Build history of the part. All positions in model axes, mm. Round coordinates to 2 decimals unless told otherwise and drop trailing zeros. Write each loop counter-clockwise with the first axis right and the second up, starting at its lowest first coordinate (ties: lowest second). Pieces come first, ordered by that corner, then holes. Notation, with made-up numbers: (-8.75, 52) - (12.25, 52) arc R23 ccw to (12.25, 82) - close; hole circle Ø6 at (55, -30.5). An arc over 180 degrees is marked (long way). Answer as a JSON object with one key per item and string values. Group by question number.
Item 1: Slice it at C-C, the plane x = -3.5. List the corners of the cut face in (y, z), then the cut area to 3 significant figures.
Item 2: Slice it at A-A, the plane z = 0. List the corners of the cut face in (x, y), then the cut area to 3 significant figures.
Item 3: Flat gauge pins, fed straight in: pin 1 (4 mm diameter, centred on x = -33.02, z = 0, fed in from -Y); pin 2 (1.5 mm diameter, centred on y = 3, z = -5.5, fed in from -X). Where does each tip first touch, or does it go through?
Item 4: Slice it at B-B, the plane z = 33.02. List the corners of the cut face in (x, y).
Item 5: Probe line 1 (X direction, y = 5.5, z = 26); line 2 (Z direction, x = 33.5, y = 0.5). List the from-to ranges inside material, lowest first. Write a range as from..to.
Item 6: Slice it at D-D, the plane y = 2.25. Give the number of separate pieces and of enclosed holes in the cut face, then the cut area to 3 significant figures.
from build123d import *

# Parameters (mm, degrees)
SKETCH1_R           = 38.1
SKETCH1_R_2         = 1.6256
BOSS_EXTRUDE1_DEPTH = 6.35


with BuildPart() as part:
    # Sketch1 → Boss-Extrude1 (new body)
    with BuildSketch(Plane(origin=(0, 0, 0), x_dir=(1, 0, 0), z_dir=(0, 1, 0))):
        with Locations(Location((0, 0, 0), (0, 0, 270))):
            Circle(SKETCH1_R)
        with Locations(Location((0, 33.02, 0), (0, 0, 270))):
            Circle(SKETCH1_R_2, mode=Mode.SUBTRACT)
        with Locations(Location((33.02, 0, 0), (0, 0, 270))):
            Circle(SKETCH1_R_2, mode=Mode.SUBTRACT)
        with Locations(Location((0, -33.02, 0), (0, 0, 270))):
            Circle(SKETCH1_R_2, mode=Mode.SUBTRACT)
        with Locations(Location((-33.02, 0, 0), (0, 0, 270))):
            Circle(SKETCH1_R_2, mode=Mode.SUBTRACT)
        with BuildLine():
            Line((29.48483871, -14.864880969), (22.32486724, -11.89912368))
            ThreePointArc((22.32486724, -11.89912368), (17.888387876, -17.888387876), (11.89912368, -22.32486724))
            Line((11.89912368, -22.32486724), (14.864880969, -29.48483871))
            ThreePointArc((14.864880969, -29.48483871), (12.636206937, -30.506502164), (10.33787126, -31.359987529))
            Line((10.33787126, -31.359987529), (7.37211397, -24.200016059))
            ThreePointArc((7.37211397, -24.200016059), (0, -25.298000744), (-7.37211397, -24.200016059))
            Line((-7.37211397, -24.200016059), (-10.33787126, -31.359987529))
            ThreePointArc((-10.33787126, -31.359987529), (-12.636206937, -30.506502164), (-14.864880969, -29.48483871))
            Line((-14.864880969, -29.48483871), (-11.89912368, -22.32486724))
            ThreePointArc((-11.89912368, -22.32486724), (-17.888387876, -17.888387876), (-22.32486724, -11.89912368))
            Line((-22.32486724, -11.89912368), (-29.48483871, -14.864880969))
            ThreePointArc((-29.48483871, -14.864880969), (-30.506502164, -12.636206937), (-31.359987529, -10.33787126))
            Line((-31.359987529, -10.33787126), (-24.200016059, -7.37211397))
            ThreePointArc((-24.200016059, -7.37211397), (-25.298000744, 0), (-24.200016059, 7.37211397))
            Line((-24.200016059, 7.37211397), (-31.359987529, 10.33787126))
            ThreePointArc((-31.359987529, 10.33787126), (-30.506502164, 12.636206937), (-29.48483871, 14.864880969))
            Line((-29.48483871, 14.864880969), (-22.32486724, 11.89912368))
            ThreePointArc((-22.32486724, 11.89912368), (-17.888387876, 17.888387876), (-11.89912368, 22.32486724))
            Line((-11.89912368, 22.32486724), (-14.864880969, 29.48483871))
            ThreePointArc((-14.864880969, 29.48483871), (-12.636206937, 30.506502164), (-10.33787126, 31.359987529))
            Line((-10.33787126, 31.359987529), (-7.37211397, 24.200016059))
            ThreePointArc((-7.37211397, 24.200016059), (0, 25.298000744), (7.37211397, 24.200016059))
            Line((7.37211397, 24.200016059), (10.33787126, 31.359987529))
            ThreePointArc((10.33787126, 31.359987529), (12.636206937, 30.506502164), (14.864880969, 29.48483871))
            Line((14.864880969, 29.48483871), (11.89912368, 22.32486724))
            ThreePointArc((11.89912368, 22.32486724), (17.888387876, 17.888387876), (22.32486724, 11.89912368))
            Line((22.32486724, 11.89912368), (29.48483871, 14.864880969))
            ThreePointArc((29.48483871, 14.864880969), (30.506502164, 12.636206937), (31.359987529, 10.33787126))
            Line((31.359987529, 10.33787126), (24.200016059, 7.37211397))
            ThreePointArc((24.200016059, 7.37211397), (25.298000744, 0), (24.200016059, -7.37211397))
            Line((24.200016059, -7.37211397), (31.359987529, -10.33787126))
            ThreePointArc((31.359987529, -10.33787126), (30.506502164, -12.636206937), (29.48483871, -14.864880969))
        make_face(mode=Mode.SUBTRACT)
    extrude(amount=BOSS_EXTRUDE1_DEPTH)


solid = part.part
Geometry says:
{
 "1": {"outline": "(0, -37.94) - (6.35, -37.94) - (6.35, -25.05) - (0, -25.05) - close; (0, 25.05) - (6.35, 25.05) - (6.35, 37.94) - (0, 37.94) - close", "area": "164 mm^2"},
 "2": {"outline": "(-38.1, 0) - (-34.65, 0) - (-34.65, 6.35) - (-38.1, 6.35) - close; (-31.39, 0) - (-25.3, 0) - (-25.3, 6.35) - (-31.39, 6.35) - close; (25.3, 0) - (31.39, 0) - (31.39, 6.35) - (25.3, 6.35) - close; (34.65, 0) - (38.1, 0) - (38.1, 6.35) - (34.65, 6.35) - close", "area": "121 mm^2"},
 "3": {"pin 1": "stops at y = 0", "pin 2": "stops at x = -37.8"},
 "4": {"outline": "(-19.01, 0) - (-1.63, 0) - (-1.63, 6.35) - (-19.01, 6.35) - close; (1.63, 0) - (19.01, 0) - (19.01, 6.35) - (1.63, 6.35) - close"},
 "5": {"line 1": "x = -27.85..-13.42, -8.12..8.12, 13.42..27.85", "line 2": "z = -18.15..-1.55, 1.55..18.15"},
 "6": {"separate pieces": "1", "enclosed holes": "5", "area": "2,210 mm^2"}
}
